Autodesk Fusion 360 part; units mm, degrees
sketch "Sketch1" plane through (0, 0, 0) normal (1, 0, 0) x (0, 0, -1)
  line L0 (0, 0) -> (-25, 0)
  line L1 (-25, 0) -> (-25, 11)
  line L2 (-25, 11) -> (-20, 11)
  line L3 (0, 5) -> (0, 0)
  line L4 (0, 0) -> (0, 5)
  line L5 (-20, 5) -> (-20, 11)
  line L6 (-20, 5) -> (0, 5)
  point P0 (0, 5)
  point P1 (-20, 11)
  point P2 (-20, 5)
  point P3 (-25, 11)
  point P4 (-25, 0)
extrude "Extrude1" add sketch "Sketch1" along normal blind 9
sketch "Sketch2" plane through (0, 0, 20) normal (0, 0, -1) x (-1, 0, 0)
  line L0 (0, 5) -> (0, 11)
  line L1 (0, 11) -> (-9, 11)
  line L2 (-9, 11) -> (-9, 5)
  line L3 (-9, 5) -> (0, 5)
  circle A0 centre (-4.5, 8) radius 2
  dimension "d9" = 4
  dimension "d11" = 4.5
sketch "Sketch3" plane through (0, 5, 0) normal (0, 1, 0) x (-1, 0, 0)
  line L0 (0, 0) -> (0, 20)
  line L1 (0, 20) -> (-9, 20)
  line L2 (-9, 20) -> (-9, 0)
  line L3 (-9, 0) -> (0, 0)
  circle A0 centre (-4.5, 9) radius 2
  dimension "d12" = 4
  dimension "d14" = 4.5
extrude "Extrude2" cut sketch "Sketch3" against normal blind 13 contours A0
extrude "Extrude3" cut sketch "Sketch2" against normal blind 11 contours A0
fillet "Fillet1" radius 2.5 1 edges at (0, 2.5, 0)
fillet "Fillet2" radius 2.5 1 edges at (9, 2.5, 0)
extrude "Extrude4" add 1 faces at (6, 11, 23.3333) along direction (0, 1, 0) blind 1
fillet "Fillet3" radius 2.5 1 edges at (0, 12, 22.5)
fillet "Fillet4" radius 2.5 1 edges at (9, 12, 22.5)
Could you check a few things on this model? Use its own coordinates, in mm. A direction names the side the tool comes from. Round coordinates to 2 decimals unless told otherwise and drop trailing zeros. Order: outer loops, then holes, each group sorted by start corner. A loop starts at its lowest first (then second) coordinate and runs counter-clockwise, first axis right, second up.
(1) Imagine slicing it at C-C (y = 8.5). Write out the boundary of the cut face in (x, z).
Response values:
outline: (0, 20) - (2.56, 20) - (2.56, 25) - (0, 25) - close; (6.44, 20) - (9, 20) - (9, 25) - (6.44, 25) - close
(2) Which directions (+Z, -Z, +X, -X, +Y, -Y) give clear straight access to the entire face, cutting with the end or side of a thin tool? Please do faces 1 (the flat face through (9, 4, 16)), 2 (the flat face through (3, 10, 20)).
Response values:
face 1: +Z, -Z, +X, +Y, -Y
face 2: -Z, +X, -X, +Y
(3) If we mould it in two halves opening along Y, with no side actions, what happens to faces 3 (the flat face through (4, 5, 25)), 4 (the flat face through (4, 0, 12)), 5 (the flat face through (6.4, 5, 10.1)), 6 (the cylindrical face through (4.76, 9.983, 22.465))? For each: released by +Y, released by -Y, zero draft, split by the parting line, or undercut.
Response values:
face 3: zero draft
face 4: released by -Y
face 5: released by +Y
face 6: undercut
(4) Please list where these lines run through material, in increasing order: line 1 along Z through (x, y) = (4.5, 3.5); line 2 along Y through (x, z) = (1.5, 17.75); line 3 along Y through (x, z) = (4.5, 23.25).
Response values:
line 1: z = 0 to 7, 11 to 25
line 2: y = 0 to 5
line 3: y = 0 to 6, 10 to 12
(5) Imagine slicing it at A-A (x = 4.5). Write out the boundary of the cut face in (y, z), plus the area to 3 significant figures.
Response values:
outline: (0, 0) - (5, 0) - (5, 7) - (0, 7) - close; (0, 11) - (5, 11) - (5, 20) - (6, 20) - (6, 25) - (0, 25) - close; (10, 20) - (12, 20) - (12, 25) - (10, 25) - close
area: 120 mm2
(6) Imagine slicing it at B-B (z = 9). Write out the boundary of the cut face in (x, y), plus the area to 3 significant figures.
Response values:
outline: (0, 0) - (2.5, 0) - (2.5, 5) - (0, 5) - close; (6.5, 0) - (9, 0) - (9, 5) - (6.5, 5) - close
area: 25.0 mm2
(7) Imagine slicing it at D-D (y = 1.75). Write out the boundary of the cut face in (x, z), plus the area to 3 significant figures.
Response values:
outline: (0, 2.5) arc R2.5 ccw to (2.5, 0) - (6.5, 0) arc R2.5 ccw to (9, 2.5) - (9, 25) - (0, 25) - close; hole circle Ø4 at (4.5, 9)
area: 210 mm2
(8) I'm going to push flat-ended pins straight in: pin 1 (1.5 mm diameter, centred on x = 3, y = 9.5, fed in from -Z); pin 2 (5 mm diameter, centred on x = 6.5, z = 8.5, fed in from +Y). Where does each tip first touch, or does it pass through?
Response values:
pin 1: stops at z = 20
pin 2: stops at y = 5
